from build123d import *

# Parameters (mm, degrees)
CUT_EXTRUDE1_DEPTH = 1.85
SKETCH4_R          = 0.9
CUT_EXTRUDE2_DEPTH = 21.003062266


with BuildPart() as part:
    # Sketch1 → Revolve1 (revolve)
    with BuildSketch(Plane.XY, mode=Mode.PRIVATE) as revolve1_sk:
        Polygon((7.5, 1), (7.5, 0), (14, 0), (14, 2.85), (11, 2.85), (11, 1), align=None)
    revolve(revolve1_sk.sketch.rotate(Axis((0, 1, 0), (0, -1, 0)), 180), axis=Axis((0, 1, 0), (0, -1, 0)))

    # Sketch2 → Cut-Extrude1 (cut)
    with BuildSketch(Plane(origin=(0, 2.85, 0), x_dir=(1, 0, 0), z_dir=(0, 1, 0))):
        with BuildLine():
            ThreePointArc((-7.267434673, -8.257384167), (-7.526619427, -8.021845174), (-7.778174593, -7.778174593))
            Line((-7.778174593, -7.778174593), (-9.899494937, -9.899494937))
            ThreePointArc((-9.899494937, -9.899494937), (-9.648834126, -10.143963722), (-9.392138077, -10.382087571))
            Line((-9.392138077, -10.382087571), (-7.267434673, -8.257384167))
        make_face()
        with BuildLine():
            Line((-9.899494937, -9.899494937), (-7.778174593, -7.778174593))
            ThreePointArc((-7.778174593, -7.778174593), (-8.021845174, -7.526619427), (-8.257384167, -7.267434673))
            Line((-8.257384167, -7.267434673), (-10.382087571, -9.392138077))
            ThreePointArc((-10.382087571, -9.392138077), (-10.143963722, -9.648834126), (-9.899494937, -9.899494937))
        make_face()
        with BuildLine():
            Line((10.382087571, -9.392138077), (8.257384167, -7.267434673))
            ThreePointArc((8.257384167, -7.267434673), (7.778174593, -7.778174593), (7.267434673, -8.257384167))
            Line((7.267434673, -8.257384167), (9.392138077, -10.382087571))
            ThreePointArc((9.392138077, -10.382087571), (9.648834126, -10.143963722), (9.899494937, -9.899494937))
            ThreePointArc((9.899494937, -9.899494937), (10.143963722, -9.648834126), (10.382087571, -9.392138077))
        make_face()
    extrude(amount=-CUT_EXTRUDE1_DEPTH, mode=Mode.SUBTRACT)

    # Sketch4 → Cut-Extrude2 (cut, through all)
    with BuildSketch(Plane(origin=(0, 2.85, 0), x_dir=(1, 0, 0), z_dir=(0, 1, 0))):
        with Locations(Location((-10.825317547, 6.25, 0), (0, 0, 180))):
            Circle(SKETCH4_R)
        with Locations(Location((10.825317547, 6.25, 0), (0, 0, 180))):
            Circle(SKETCH4_R)
        with Locations(Location((0, -12.5, 0), (0, 0, 180))):
            Circle(SKETCH4_R)
    extrude(amount=-CUT_EXTRUDE2_DEPTH, mode=Mode.SUBTRACT)


solid = part.part
Read the model definition and answer for the solid it produces. Units are mm, in the model's axes. A direction names the side the tool comes from. Round coordinates to 2 decimals unless told otherwise and drop trailing zeros. Order: outer loops, then holes, each group sorted by start corner. A loop starts at its lowest first (then second) coordinate and runs counter-clockwise, first axis right, second up.
1) The part is cut by section C-C on z = 0. Write down the section's boundary in (x, y).
2) For faces 4 (the face through (-2, 2.85, -11)), 5 (the face through (0, 2, -11)), determine the directions among +Z, -Z, +X, -X, +Y, -Y from which every point of the face is accessible in a straight line to the end or side of a thin tool.
3) Flat-ended cylindrical pins translate along their axes: pin 1 (1 mm diameter, centred on y = 1.5, z = 7.5, fed in from +X); pin 2 (6.5 mm diameter, centred on x = -4, z = 4.5, fed in from +Y). Find the tip coordinate at first contact, or state that the pin passes through.
4) The part is cut by section A-A on y = 2.5. Write down the section's boundary in (x, z), plus the area to 3 significant figures.
5) The mould has two halves that part along X. Classify faces 1 (the face through (2, 2.85, 12)), 2 (the face through (-12.932, 1.445, 5.362)), 3 (the face through (9.33, 1.94, 8.34)): released by +X, released by -X, zero draft, split by the parting line, or undercut.
6) Straight lines are drawn through the part: L1, parallel to Z at x = -8.5, y = 2; L2, parallel to Y at x = 3.75, z = 9.75; L3, parallel to X at y = 2.4, z = -4.5. For each, find the intervals that lie inside material, in ascending order.
7) The part is cut by section B-B on x = 0. Write down the section's boundary in (y, z).
8) The part is cut by section D-D on z = -6.25. Write down the section's boundary in (x, y), plus the area to 3 significant figures.
Resolved:
1. outline: (-14, 0) - (-7.5, 0) - (-7.5, 1) - (-11, 1) - (-11, 2.85) - (-14, 2.85) - close; (7.5, 0) - (14, 0) - (14, 2.85) - (11, 2.85) - (11, 1) - (7.5, 1) - close
2. face 4: +Z, -Z, +X, -X, +Y
2. face 5: +Y
3. pin 1: stops at x = 12.12
3. pin 2: stops at y = 1
4. outline: (-10.38, 9.39) arc R14 ccw (long way) to (10.38, 9.39) - (8.26, 7.27) arc R11 cw (long way) to (-8.26, 7.27) - close; (-9.39, 10.38) - (-7.27, 8.26) arc R11 cw to (7.27, 8.26) - (9.39, 10.38) arc R14 ccw to start; hole circle Ø1.8 at (-10.83, -6.25); hole circle Ø1.8 at (0, 12.5); hole circle Ø1.8 at (10.83, -6.25)
4. area: 220 mm2
5. face 1: zero draft
5. face 2: split by the parting line
5. face 3: undercut
6. L1: z = -11.12 to -6.98, 6.98 to 7.51, 9.49 to 11.12
6. L2: y = 0 to 1
6. L3: x = -13.26 to -10.04, 10.04 to 13.26
7. outline: (0, -14) - (2.85, -14) - (2.85, -11) - (1, -11) - (1, -7.5) - (0, -7.5) - close; (0, 7.5) - (1, 7.5) - (1, 11) - (2.85, 11) - (2.85, 11.6) - (0, 11.6) - close; (0, 13.4) - (2.85, 13.4) - (2.85, 14) - (0, 14) - close
8. outline: (-12.53, 0) - (-11.73, 0) - (-11.73, 2.85) - (-12.53, 2.85) - close; (-9.93, 0) - (-4.15, 0) - (-4.15, 1) - (-9.05, 1) - (-9.05, 2.85) - (-9.93, 2.85) - close; (4.15, 0) - (9.93, 0) - (9.93, 2.85) - (9.05, 2.85) - (9.05, 1) - (4.15, 1) - close; (11.73, 0) - (12.53, 0) - (12.53, 2.85) - (11.73, 2.85) - close
8. area: 19.4 mm2
